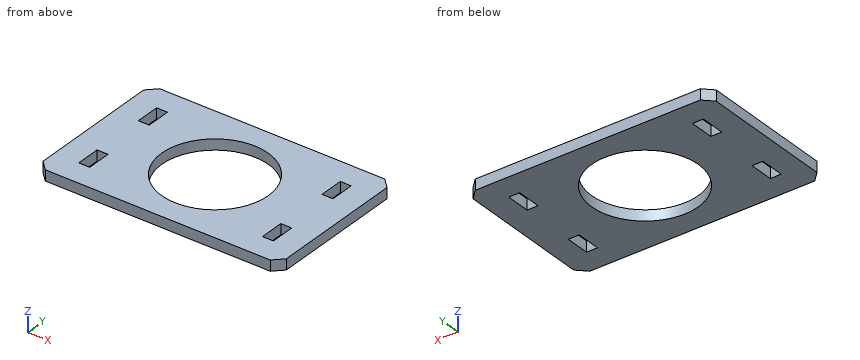
```python
from build123d import *

# Parameters (mm, degrees)
F0_W     = 400
F0_H     = 250
F0_W_2   = 18
F0_H_2   = 40
F0_R     = 87.5
F1_DEPTH = 17.5
F2_SIZE  = 15


with BuildPart() as f1:
    # F0 (on Top) → F1 (new body)
    with BuildSketch(Plane.XY):
        with Locations((-107.214418, 42.974777)):
            Rectangle(F0_W, F0_H)
        with Locations((-258.214418, -22.025223)):
            Rectangle(F0_W_2, F0_H_2, mode=Mode.SUBTRACT)
        with Locations((43.785582, -22.025223)):
            Rectangle(F0_W_2, F0_H_2, mode=Mode.SUBTRACT)
        with Locations((-107.214418, 42.974777)):
            Circle(F0_R, mode=Mode.SUBTRACT)
        with Locations((-258.214418, 107.974777)):
            Rectangle(F0_W_2, F0_H_2, mode=Mode.SUBTRACT)
        with Locations((43.785582, 107.974777)):
            Rectangle(F0_W_2, F0_H_2, mode=Mode.SUBTRACT)
    extrude(amount=F1_DEPTH)

    # F2
    f2_edges = [f1.edges().sort_by_distance(p)[0] for p in [
        (-307.214418, 167.974777, 8.75),
        (92.785582, 167.974777, 8.75),
        (92.785582, -82.025223, 8.75),
        (-307.214418, -82.025223, 8.75),
    ]]
    chamfer(f2_edges, length=F2_SIZE)


solid = f1.part
```
Source: CAD feature listing. Evaluate the final solid. Frame: model axes, mm. Round coordinates to 2 decimals unless told otherwise and drop trailing zeros. Loops run counter-clockwise (first coordinate to the right, second up) from the corner with the lowest first, then second, coordinate; pieces in that order, holes last. Notation, with made-up numbers: M -36.75,-23.75 L -30.75,-23.75 A23 cw -30.75,-11.75 Z; hole C 23,39 d7. An arc over 180 degrees is marked long. Use a Markdown table: item, result. Add a question column.
1. Ray query, line 1 along Y through (x, z) = (39, 12); line 2 along Y through (x, z) = (-128, 7); line 3 along X through (y, z) = (37, 5). Return the intervals inside material, ascending. Write a range as [from, to].
2. Cut plane C-C, the plane y = -12. Output: boundary loops of the cut face in (x, z), and give its area (3 significant figures).
3. Cut plane B-B, the plane y = 78. Output: boundary loops of the cut face in (x, z), and give its area (3 significant figures).
4. Cut plane A-A, the plane x = -53.5. Output: boundary loops of the cut face in (y, z).
5. Cut plane D-D, the plane z = 6.75. Output: boundary loops of the cut face in (x, y).
Solution:
| question | item | result |
|---|---|---|
| 1 | line 1 | y = [-82.03, -42.03], [-2.03, 87.97], [127.97, 167.97] |
| 1 | line 2 | y = [-82.03, -42.02], [127.97, 167.97] |
| 1 | line 3 | x = [-307.21, -194.51], [-19.92, 92.79] |
| 2 | outline | M -307.21,0 L -267.21,0 L -267.21,17.5 L -307.21,17.5 Z; M -249.21,0 L -175.29,0 L -175.29,17.5 L -249.21,17.5 Z; M -39.14,0 L 34.79,0 L 34.79,17.5 L -39.14,17.5 Z; M 52.79,0 L 92.79,0 L 92.79,17.5 L 52.79,17.5 Z |
| 2 | area | 3,990 mm2 |
| 3 | outline | M -307.21,0 L -187.4,0 L -187.4,17.5 L -307.21,17.5 Z; M -27.03,0 L 92.79,0 L 92.79,17.5 L -27.03,17.5 Z |
| 3 | area | 4,190 mm2 |
| 4 | outline | M -82.03,0 L -26.1,0 L -26.1,17.5 L -82.03,17.5 Z; M 112.05,0 L 167.97,0 L 167.97,17.5 L 112.05,17.5 Z |
| 5 | outline | M -307.21,-67.03 L -292.21,-82.03 L 77.79,-82.03 L 92.79,-67.03 L 92.79,152.97 L 77.79,167.97 L -292.21,167.97 L -307.21,152.97 Z; hole M -267.21,-42.03 L -249.21,-42.03 L -249.21,-2.03 L -267.21,-2.03 Z; hole M -267.21,87.97 L -249.21,87.97 L -249.21,127.97 L -267.21,127.97 Z; hole C -107.21,42.97 d175; hole M 34.79,-42.03 L 52.79,-42.03 L 52.79,-2.03 L 34.79,-2.03 Z; hole M 34.79,87.97 L 52.79,87.97 L 52.79,127.97 L 34.79,127.97 Z |
